from build123d import *

# Parameters (mm, degrees)
SKETCH1_W                                       = 200
SKETCH1_H                                       = 400
BOSS_EXTRUDE1_DEPTH                             = 15
CSK_FOR_M4_FLAT_HEAD_MACHINE_SCREW1_D           = 4.3
CSK_FOR_M4_FLAT_HEAD_MACHINE_SCREW1_CSINK_D     = 9.4
CSK_FOR_M4_FLAT_HEAD_MACHINE_SCREW1_CSINK_ANGLE = 90
M4X0_7_TAPPED_HOLE1_D                           = 3.3


with BuildPart() as part:
    # Sketch1 → Boss-Extrude1 (new body)
    with BuildSketch(Plane.XY):
        Rectangle(SKETCH1_W, SKETCH1_H)
    extrude(amount=BOSS_EXTRUDE1_DEPTH)

    # CSK for M4 Flat Head Machine Screw1 (through all)
    with Locations(Plane.XY.offset(15)):
        with Locations((-77.5, -160), (-52.5, -160), (-52.5, -190), (-77.5, -190), (52.5, -160), (77.5, -160), (77.5, -190), (52.5, -190)):
            CounterSinkHole(CSK_FOR_M4_FLAT_HEAD_MACHINE_SCREW1_D / 2, CSK_FOR_M4_FLAT_HEAD_MACHINE_SCREW1_CSINK_D / 2, counter_sink_angle=CSK_FOR_M4_FLAT_HEAD_MACHINE_SCREW1_CSINK_ANGLE)

    # M4x0.7 Tapped Hole1 (through all)
    with Locations(Plane.XY.offset(15)):
        with Locations((-34.5, -190.5), (34.5, -190.5), (-34.5, -130.5), (34.5, -130.5), (-34.5, -70.5), (34.5, -70.5), (-34.5, -10.5), (34.5, -10.5), (-34.5, 49.5), (34.5, 49.5), (-34.5, 109.5), (34.5, 109.5), (-34.5, 169.5), (34.5, 169.5)):
            Hole(M4X0_7_TAPPED_HOLE1_D / 2)


solid = part.part
Verification items for the finished model (mm, model axes). Coordinates: 2 decimals unless noted, no trailing zeros. Write each question's results on one line, items separated by ' | '.
1) Gauge pin test, flat ends, axial feed: pin 1 Ø2.5 at (x, y) = (34.5, -10.5) entering from -Z; pin 2 Ø5.5 at (x, y) = (-77.5, -160) entering from +Z. Record the tip position at first contact, or that the pin passes through.
Solved:
pin 1: passes through | pin 2: stops at z = 13.05
2) Scan lines: line 1 along X through (y, z) = (109.5, 6.75); line 2 along Y through (x, z) = (-52.5, 6.75). Record each from-to range of solid material in increasing order. Write a range as [from, to].
Solved:
line 1: x = [-100, -36.15], [-32.85, 32.85], [36.15, 100] | line 2: y = [-200, -192.15], [-187.85, -162.15], [-157.85, 200]
3) Release check for a two-part mould opening along X. For faces 1 (the face through (-1, 3, 0)), 2 (the face through (100, -3, 7)), 3 (the face through (50.331, -159.317, 12.574)) record: pulls with the +X half, pulls with the -X half, needs draft (parallel to the pull), parting line crosses it, or undercut.
Solved:
face 1: needs draft | face 2: pulls with the +X half | face 3: undercut
